from build123d import *
from OCP.BRepFilletAPI import BRepFilletAPI_MakeChamfer

# Parameters (mm, degrees)
SKETCH1_R                = 1.65
BOSS_EXTRUDE1_DEPTH      = 20
SKETCH3_R                = 1.65
CUT_EXTRUDE3_DEPTH       = 39.673925324
CUT_EXTRUDE4_DEPTH       = 12
CUT_EXTRUDE5_START       = -4
CUT_EXTRUDE5_DEPTH       = 14.65
CUT_EXTRUDE11_DEPTH      = 42.915062925
CUT_EXTRUDE11_DEPTH_BACK = 42.915062925
CUT_EXTRUDE10_DEPTH      = 5
CUT_EXTRUDE10_DEPTH_BACK = 39.898875305
SKETCH10_W               = 9.115200733
SKETCH10_H               = 9.576012389
CUT_EXTRUDE7_DEPTH       = 4.5
CUT_EXTRUDE8_DEPTH       = 36.587532929
CUT_EXTRUDE8_DEPTH_BACK  = 36.587532929
SKETCH8_R                = 1.65
CUT_EXTRUDE9_START       = 2
SKETCH9_R                = 3.5
CUT_EXTRUDE9_DEPTH       = 34.587532929
CHAMFER6_SIZE            = 1.8
CUT_EXTRUDE12_DEPTH      = 39.673925324
CHAMFER7_SIZE            = 0.3
CHAMFER7_SIZE2           = 0.219615242
CUT_EXTRUDE13_DEPTH      = 42.915062925
SKETCH14_R               = 3.1
CUT_EXTRUDE14_DEPTH      = 1.8
CHAMFER8_START           = -4.6500001
CHAMFER8_OUTLINE_R       = 3.1
CHAMFER8_DEPTH           = 1.8000001
CHAMFER8_START_2         = -4.65
CHAMFER8_3_DEPTH         = 1.8
FILLET1_R                = 3


with BuildPart() as part:
    # Sketch1 → Boss-Extrude1 (new body)
    with BuildSketch(Plane.XY):
        with BuildLine():
            Line((-3.894375, -2.540933561), (-2.7, -4.371498599))
            ThreePointArc((-2.7, -4.371498599), (2.076657931, -7.765356095), (7.885150706, -6.993254178))
            ThreePointArc((7.885150706, -6.993254178), (12.369935761, -5.200285461), (17.161085198, -4.589612979))
            Line((17.161085198, -4.589612979), (29.253037683, -4.589612979))
            ThreePointArc((29.253037683, -4.589612979), (34.634878658, -0.374699645), (30, 4.65))
            Line((30, 4.65), (26, 4.65))
            Line((26, 4.65), (26, 12.5))
            Line((26, 12.5), (-4.65, 12.5))
            Line((-4.65, 12.5), (-4.65, 0))
            ThreePointArc((-4.65, 0), (-4.457092312, -1.325453932), (-3.894375, -2.540933561))
        make_face()
        Circle(SKETCH1_R, mode=Mode.SUBTRACT)
        with Locations((30, 0)):
            Circle(SKETCH1_R, mode=Mode.SUBTRACT)
    extrude(amount=BOSS_EXTRUDE1_DEPTH)

    # Sketch3 → Cut-Extrude3 (cut, through all)
    with BuildSketch(Plane(origin=(26, 0, 0), x_dir=(0, 0, -1), z_dir=(1, 0, 0))):
        with Locations(Location((-16, 7.6, 0), (0, 0, 90))):
            Circle(SKETCH3_R)
    extrude(amount=-CUT_EXTRUDE3_DEPTH, mode=Mode.SUBTRACT)

    # Sketch4 → Cut-Extrude4 (cut)
    with BuildSketch(Plane(origin=(0, 0, 0), x_dir=(-1, 0, 0), z_dir=(0, 0, -1))):
        Polygon((1.58771324, -2.75), (6.896922601, -2.75), (6.896922601, 2.75), (1.58771324, 2.75), (-1.58771324, 2.75), (-3.175426481, 0), (-1.58771324, -2.75), align=None)
    extrude(amount=-CUT_EXTRUDE4_DEPTH, mode=Mode.SUBTRACT)

    # Sketch5 → Cut-Extrude5 (cut)
    with BuildSketch(Plane(origin=(26, 0, 0), x_dir=(0, 0, -1), z_dir=(1, 0, 0)).offset(CUT_EXTRUDE5_START)):
        Polygon((-13.3, 6.041154273), (0, 6.041154273), (0, 12.5), (-20, 13.02709253), (-20, 6.791709623), (-16, 4.482308546), align=None)
    extrude(amount=-CUT_EXTRUDE5_DEPTH, mode=Mode.SUBTRACT)

    # Sketch11 → Cut-Extrude11 (cut, two sides: drawn at the far end of the back side and taken through both)
    with BuildSketch(Plane(origin=(0, 0, 0), x_dir=(1, 0, 0), z_dir=(0, 1, 0)).offset(-CUT_EXTRUDE11_DEPTH_BACK)):
        Polygon((22, 0), (-4.65, -10), (-4.65, 0), align=None)
    extrude(amount=CUT_EXTRUDE11_DEPTH + CUT_EXTRUDE11_DEPTH_BACK, mode=Mode.SUBTRACT)

    # Sketch10 → Cut-Extrude10 (cut, two sides: drawn at the far end of the back side and taken through both)
    with BuildSketch(Plane.XY.offset(7.5).offset(-CUT_EXTRUDE10_DEPTH_BACK)):
        with Locations((30.557600367, -0.138006194)):
            Rectangle(SKETCH10_W, SKETCH10_H)
    extrude(amount=CUT_EXTRUDE10_DEPTH + CUT_EXTRUDE10_DEPTH_BACK, mode=Mode.SUBTRACT)

    # Sketch7 → Cut-Extrude7 (cut)
    with BuildSketch(Plane(origin=(0, 0, 12.5), x_dir=(-1, 0, 0), z_dir=(0, 0, -1))):
        Polygon((-27.2, -1.616580754), (-27.2, 1.616580754), (-30, 3.233161507), (-32.8, 1.616580754), (-32.8, -1.616580754), (-30, -3.233161507), align=None)
    extrude(amount=-CUT_EXTRUDE7_DEPTH, mode=Mode.SUBTRACT)

    # Sketch8 → Cut-Extrude8 (cut, two sides: drawn at the far end of the back side and taken through both)
    with BuildSketch(Plane.ZY.offset(-22).offset(-CUT_EXTRUDE8_DEPTH_BACK)):
        with Locations((4, 0)):
            Circle(SKETCH8_R)
        with BuildLine():
            Line((12.5, 12.5), (0, 12.5))
            Line((0, 12.5), (0, 0))
            ThreePointArc((0, 0), (3.661165235, 8.838834765), (12.5, 12.5))
        make_face()
    extrude(amount=CUT_EXTRUDE8_DEPTH + CUT_EXTRUDE8_DEPTH_BACK, mode=Mode.SUBTRACT)

    # Sketch9 → Cut-Extrude9 (cut, through all)
    with BuildSketch(Plane.ZY.offset(-22).offset(CUT_EXTRUDE9_START)):
        with Locations((4, 0)):
            Circle(SKETCH9_R)
    extrude(amount=CUT_EXTRUDE9_DEPTH, mode=Mode.SUBTRACT)

    # Chamfer6
    # the kernel refuses this chamfer: 1.8 mm, written as the material it takes off along each edge
    with BuildSketch(Plane(origin=(20, 0, 4), x_dir=(0, 0, 1), z_dir=(0, -1, 0))) as chamfer6_piece_1:
        Polygon((1.65, -CHAMFER6_SIZE), (1.65 + CHAMFER6_SIZE, 0), (1.65, 0), align=None)
    revolve(axis=Axis((20, 0, 4), (-1, 0, 0)), mode=Mode.SUBTRACT)

    # Sketch12 → Cut-Extrude12 (cut, through all)
    with BuildSketch(Plane(origin=(26, 0, 0), x_dir=(0, 0, -1), z_dir=(1, 0, 0))):
        Polygon((-4, 0), (-2.833273811, -1.166726189), (-2.03, -0.363452378), (-2.03, 0.363452378), (-2.833273811, 1.166726189), align=None)
        Polygon((-16, 7.6), (-14.833273811, 6.433273811), (-14.03, 7.236547622), (-14.03, 7.963452378), (-14.833273811, 8.766726189), align=None)
    extrude(amount=-CUT_EXTRUDE12_DEPTH, mode=Mode.SUBTRACT)

    # Chamfer7: one chamfer whose edges measure the first distance from different faces: ONE call of the kernel's chamfer builder (chamfer() names one face for all edges)
    chamfer7_edges_1 = [part.edges().sort_by_distance(p)[0] for p in [
        (-4.457092312, -1.325453932, 20),
        (-3.2971875, -3.45621608, 20),
        (2.076657931, -7.765356095, 20),
        (12.369935761, -5.200285461, 20),
        (23.207061441, -4.589612979, 20),
        (34.634878658, -0.374699645, 20),
        (-1.65, 0, 20),
        (28, 4.65, 20),
        (28.35, 0, 20),
        (26, 8.575, 20),
        (24, 12.5, 20),
        (-4.65, 6.25, 20),
        (1.35, 12.5, 20),
        (22, 9.645854812, 20),
        (7.35, 9.645854812, 20),
    ]]
    chamfer7_edges_2 = [part.edges().sort_by_distance(p)[0] for p in [
        (14.675, 6.791709623, 20),
    ]]
    chamfer7_side_2 = [part.faces().sort_by_distance(p)[0] for p in [
        (12.200528513, 2.041085784, 20),
    ]]
    chamfer7 = BRepFilletAPI_MakeChamfer(part.part.solid().wrapped)
    for e in chamfer7_edges_1:
        chamfer7.Add(CHAMFER7_SIZE, e.wrapped)
    for e in chamfer7_edges_2:
        chamfer7.Add(CHAMFER7_SIZE, CHAMFER7_SIZE2, e.wrapped, chamfer7_side_2[0].wrapped)  # the first distance lies on this face
    add(Compound.cast(chamfer7.Shape()), mode=Mode.REPLACE)

    # Sketch13 → Cut-Extrude13 (cut, through all)
    with BuildSketch(Plane.XY.offset(20)):
        with BuildLine():
            Line((2.668200105, 13.768506402), (3.468200105, 13.768506402))
            Line((3.468200105, 13.768506402), (3.468200105, 5.400266455))
            ThreePointArc((3.468200105, 5.400266455), (6.363895276, 0.831941508), (4.739860969, -4.327240201))
            ThreePointArc((4.739860969, -4.327240201), (4, -6), (3.260139031, -4.327240201))
            ThreePointArc((3.260139031, -4.327240201), (5.406317163, 0.353905339), (2.668200105, 4.715317853))
            Line((2.668200105, 4.715317853), (0.468200105, 13.768506402))
            Line((0.468200105, 13.768506402), (2.668200105, 13.768506402))
        make_face()
    extrude(amount=-CUT_EXTRUDE13_DEPTH, mode=Mode.SUBTRACT)

    # Sketch14 → Cut-Extrude14 (cut)
    with BuildSketch(Plane.ZY.offset(4.65)):
        with Locations(Location((16, 7.6, 0), (0, 0, 270))):
            Circle(SKETCH14_R)
    extrude(amount=-CUT_EXTRUDE14_DEPTH, mode=Mode.SUBTRACT)

    # Chamfer8: read off the stored shape, not the designer's step
    # Chamfer8 outline → Chamfer8 (add)
    with BuildSketch(Plane.YZ.offset(CHAMFER8_START)):
        with Locations((7.6, 16)):
            Circle(CHAMFER8_OUTLINE_R)
    extrude(amount=CHAMFER8_DEPTH)

    # Chamfer8 2 outline → Chamfer8 2 (revolve, cut)
    with BuildSketch(Plane(origin=(0, 7.6, 16), x_dir=(0, 1, 0), z_dir=(0, 0, -1))):
        Polygon((0, -4.65), (3.1, -4.65), (1.64999615, -3.19999615), (0, -3.19999615), align=None)
    revolve(axis=Axis((0, 7.6, 16), (1, 0, 0)), mode=Mode.SUBTRACT)

    # Chamfer8 3 outline → Chamfer8 3 (cut)
    with BuildSketch(Plane.YZ.offset(CHAMFER8_START_2)):
        with BuildLine():
            ThreePointArc((8.766726189, 14.833273811), (7.6, 17.65), (6.433273811, 14.833273811))
            Line((6.433273811, 14.833273811), (7.236547622, 14.03))
            Line((7.236547622, 14.03), (7.963452378, 14.03))
            Line((7.963452378, 14.03), (8.766726189, 14.833273811))
        make_face()
    extrude(amount=CHAMFER8_3_DEPTH, mode=Mode.SUBTRACT)

    # Fillet1
    # the kernel refuses this fillet: 3 mm, written as the material it takes off along each edge
    with BuildSketch(Plane(origin=(3.468200105, 5.400266455, 23.613279493), x_dir=(0.7875480221604082, -0.616253286231586, 0), z_dir=(0, 0, -1))) as fillet1_piece_1:
        with BuildLine():
            CenterArc((1.471965922, -2.987012306), FILLET1_R, 95.333346889, 46.623610266)
            Line((-0.890678145, -1.138252447), (0, 0))
            ThreePointArc((0, 0), (0.596557816, -0.027785198), (1.193115632, 0))
        make_face()
    extrude(amount=20.272787919, mode=Mode.SUBTRACT)


solid = part.part
Geometry check sheet. Reference: the model listing, model coordinates, mm. A direction names the side the tool comes from. Coordinates: 2 decimals unless noted, no trailing zeros. Order: outer loops, then holes, each group sorted by start corner. A loop starts at its lowest first (then second) coordinate and runs counter-clockwise, first axis right, second up. Notation, with made-up numbers: (-16.75, -36.5) -> (29.25, -36.5) arc R35 ccw to (29.25, 0.5) -> close; hole circle Ø9 at (80, 59). An arc over 180 degrees is marked (long way). Use a Markdown table: item, result. Add a question column.
1. Mould release check, pull along Z, two halves, no side actions. Record for faces 1 (the face through (5.436, 12.155, 9.584)), 2 (the face through (28.35, 0.07, 18.33)), 3 (the face through (23.93, -0.05, 5.65)), 4 (the face through (-4.28, -1.26, 19.89)): pulls with the +Z half, pulls with the -Z half, needs draft (parallel to the pull), parting line crosses it, or undercut.
2. Set-up check for faces 5 (the face through (14.6, -0.1, 7.5)), 6 (the face through (23.755, -0.771, 2.437)), 7 (the face through (6.41, 0.31, 13.14)), 8 (the face through (14.779, 5.598, 17.932)), 9 (the face through (27.2, 0, 15)): record each of +Z, -Z, +X, -X, +Y, -Y from which the full face is reachable in a straight line by a thin tool's end or side.
3. Cross-section at A-A (x = 4). Enter the section's corners in (y, z), and give its area (3 significant figures).
4. Material ranges on L1, parallel to X at y = 0, z = 18.4; L2, parallel to X at y = 8.25, z = 18; L3, parallel to Y at x = 4, z = 13.25, recorded low to high.
5. Cross-section at B-B (z = 4). Enter the section's corners in (x, y), and give its area (3 significant figures).
6. Go/stop test with flat-tipped pins: pin 1 Ø2 at (x, z) = (29, 17) entering from +Y; pin 2 Ø1 at (y, z) = (10, 8.5) entering from +X; pin 3 Ø9.5 at (x, y) = (28.5, 2) entering from -Z; pin 4 Ø3 at (x, z) = (20, 9.5) entering from +Y. Record where each tip stops, or that it passes through.
7. Cross-section at D-D (x = 0). Give the number of separate pieces and of enclosed holes in the cut face, and give its area (3 significant figures).
Filled sheet:
| question | item | result |
|---|---|---|
| 1 | face 1 | pulls with the -Z half |
| 1 | face 2 | needs draft |
| 1 | face 3 | undercut |
| 1 | face 4 | pulls with the +Z half |
| 2 | face 5 | -X |
| 2 | face 6 | +X, -X |
| 2 | face 7 | +Z, -Z |
| 2 | face 8 | +Y |
| 2 | face 9 | -Z |
| 3 | outline | (-8, 6.75) -> (-6, 6.75) -> (-6, 20) -> (-7.7, 20) -> (-8, 19.7) -> close; (-3.65, 6.75) -> (-2.16, 6.75) arc R3.5 cw to (2.16, 6.75) -> (3.65, 6.75) -> (3.65, 20) -> (-3.65, 20) -> close; (5.14, 6.75) -> (11.1, 6.75) arc R12.5 ccw to (12.5, 12.5) -> (12.5, 19.7) -> (12.2, 20) -> (5.14, 20) -> close; hole (6.43, 14.83) -> (7.24, 14.03) -> (7.96, 14.03) -> (8.77, 14.83) arc R1.65 ccw (long way) to start |
| 3 | area | 207 mm2 |
| 4 | L1 | -4.65 to -1.65, 1.65 to 5.42, 6.42 to 28.35, 31.65 to 34.65 |
| 4 | L2 | -3.65 to 1.81, 3.47 to 7.35, 22 to 26 |
| 4 | L3 | -8 to -6, -3.65 to 3.65, 5.14 to 12.5 |
| 5 | outline | (11.34, -5.5) arc R19.1 cw to (17.16, -4.59) -> (26, -4.59) -> (26, -1.65) -> (21.8, -1.65) -> (20, -3.45) -> (20, -3.5) -> (11.34, -3.5) -> close; (11.34, 3.5) -> (20, 3.5) -> (20, 3.45) -> (21.8, 1.65) -> (26, 1.65) -> (26, 9.17) -> (22, 9.17) -> (22, 6.04) -> (11.34, 6.04) -> close |
| 5 | area | 86.4 mm2 |
| 6 | pin 1 | y = 4.65 |
| 6 | pin 2 | x = 26 |
| 6 | pin 3 | z = 0 |
| 6 | pin 4 | y = 6.04 |
| 7 | separate pieces | 2 |
| 7 | enclosed holes | 1 |
| 7 | area | 171 mm2 |
